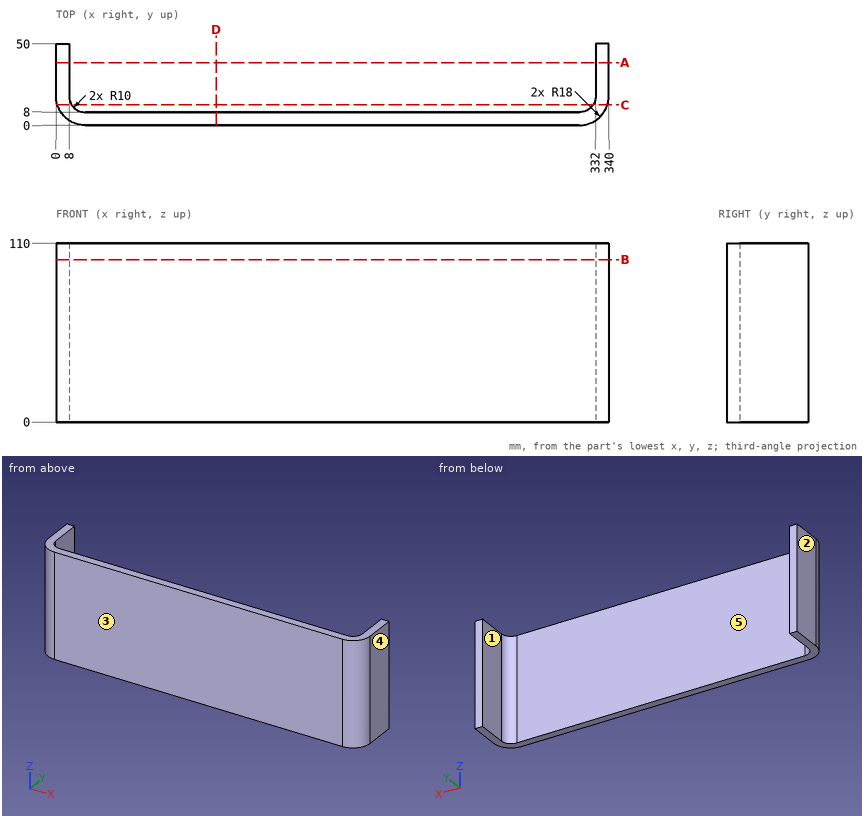
Could you check a few things on this drawing? It's one solid part, dimensions in mm from its lowest x, y, z. A direction names the side the tool comes from. Round coordinates to 2 decimals unless told otherwise and drop trailing zeros. Write each loop counter-clockwise with the first axis right and the second up, starting at its lowest first coordinate (ties: lowest second). Pieces come first, ordered by that corner, then holes. Notation, with made-up numbers: (5.25, 55) -> (13.25, 55) arc R11 ccw to (13.25, 59) -> close; hole circle Ø3 at (26.25, 81). An arc over 180 degrees is marked (long way). One line per question, with ' | ' between items. Start each with the question number.
1) Suppose I cut it at C-C on y = 12.5. Write out the boundary of the cut face in (x, z), then the cut area to 3 significant figures.
2) I'm going to push flat-ended pins straight in: P1, Ø12, axis at x = 285, z = 49.5, coming from the +Y side; P2, Ø4, axis at y = 9.5, z = 67, coming from the -X side. Where does each tip first touch, or does it pass through?
3) Suppose I cut it at A-A on y = 38.5. Write out the boundary of the cut face in (x, z), then the cut area to 3 significant figures.
4) If we mould it in two halves opening along X, with no side actions, what happens to the marked faces 1, 2 and 3? For each: released by +X, released by -X, zero draft, split by the parting line, or undercut.
5) I need wall thicknesses on line 1 (X direction, y = 45, z = 97); line 2 (Y direction, x = 282, z = 90); line 3 (X direction, y = 14, z = 6). Which ranges of each line are inside material? Lowest first, please. Write a range as [from, to].
6) Suppose I cut it at D-D on x = 98.5. Write out the boundary of the cut face in (y, z), then the cut area to 3 significant figures.
7) On a 3-axis mill with a long thin cutter (end or side, diameter ignored), from which of +Z, -Z, +X, -X, +Y, -Y can I reach the whole of each face in a straight line? I mean the marked faces 4 and 5. Say none if no direction works.
8) Suppose I cut it at B-B on z = 100. Write out the boundary of the cut face in (x, y).
Return value:
1) outline: (0.86, 0) -> (9.65, 0) -> (9.65, 110) -> (0.86, 110) -> close; (330.35, 0) -> (339.14, 0) -> (339.14, 110) -> (330.35, 110) -> close | area: 1,930 mm2
2) P1: stops at y = 8 | P2: stops at x = 1.21
3) outline: (0, 0) -> (8, 0) -> (8, 110) -> (0, 110) -> close; (332, 0) -> (340, 0) -> (340, 110) -> (332, 110) -> close | area: 1,760 mm2
4) face 1: undercut | face 2: released by -X | face 3: zero draft
5) line 1: x = [0, 8], [332, 340] | line 2: y = [0, 8] | line 3: x = [0.45, 8.83], [331.17, 339.55]
6) outline: (0, 0) -> (8, 0) -> (8, 110) -> (0, 110) -> close | area: 880 mm2
7) face 4: +Z, -Z, +X, +Y, -Y | face 5: +Z, -Z, +Y
8) outline: (0, 18) arc R18 ccw to (18, 0) -> (322, 0) arc R18 ccw to (340, 18) -> (340, 50) -> (332, 50) -> (332, 18) arc R10 cw to (322, 8) -> (18, 8) arc R10 cw to (8, 18) -> (8, 50) -> (0, 50) -> close
